```python
from build123d import *

# Parameters (mm, degrees)
BOSS_EXTRUDE1_DEPTH = 3.175
SKETCH2_R           = 1.5875
CUT_EXTRUDE1_DEPTH  = 64.286370995


with BuildPart() as part:
    # Sketch1 → Boss-Extrude1 (new body)
    with BuildSketch(Plane.XY):
        Polygon((40.909912505, -35.06563929), (40.909912505, -9.66563929), (-22.590087495, 41.13436071), (-47.990087495, 41.13436071), (-47.990087495, -35.06563929), align=None)
    extrude(amount=BOSS_EXTRUDE1_DEPTH)

    # Sketch2 → Cut-Extrude1 (cut, through all)
    with BuildSketch(Plane(origin=(0, 0, 0), x_dir=(-1, 0, 0), z_dir=(0, 0, -1))):
        with Locations((35.290087495, -22.36563929)):
            Circle(SKETCH2_R)
        with Locations((35.290087495, -3.31563929)):
            Circle(SKETCH2_R)
        with Locations((35.290087495, 15.73436071)):
            Circle(SKETCH2_R)
        with Locations((35.290087495, 34.78436071)):
            Circle(SKETCH2_R)
        with Locations((10.494914026, -22.36563929)):
            Circle(SKETCH2_R)
        with Locations((-8.555085974, -22.36563929)):
            Circle(SKETCH2_R)
        with Locations((-27.605085974, -22.36563929)):
            Circle(SKETCH2_R)
    extrude(amount=-CUT_EXTRUDE1_DEPTH, mode=Mode.SUBTRACT)


solid = part.part
```
Could you check a few things on this model? Use its own coordinates, in mm. Round coordinates to 2 decimals unless told otherwise and drop trailing zeros. Loops run counter-clockwise (first coordinate to the right, second up) from the corner with the lowest first, then second, coordinate; pieces in that order, holes last. Notation, with made-up numbers: M 11,82 L 37,82 A11 cw 37,103 Z; hole C 13.5,-8.5 d2. An arc over 180 degrees is marked long. Answer as CSV lines item,"result".
1) We'd pull the mould along X, two halves only. Please class faces 1 (the flat face through (40.91, -23, 2)), 2 (the cylindrical face through (8.899, -23.915, 1.565)), 3 (the flat face through (-4, -35.066, 2)), 4 (the cylindrical face through (-34.03, -4.28, 1.57)): released by +X, released by -X, zero draft, split by the parting line, or undercut.
From the geometry:
face 1,"released by +X"
face 2,"undercut"
face 3,"zero draft"
face 4,"undercut"
2) For pin 1 Ø3.5 at (x, y) = (-35.29, 34.78) entering from -Z, with a flat end and sliding along its axis, tell me the tip position at first contact or that it passes through.
From the geometry:
pin 1,"z = 0"
3) If I drill on probe 1 along Y at (x, z) = (-36, 2); probe 2 along Y at (x, z) = (29, 0.3); probe 3 along X at (y, z) = (33.5, 0.25), over which ranges is the centre line in solid material (lowest first)?
From the geometry:
probe 1,"-35.07 to -23.79, -20.95 to -4.74, -1.9 to 14.31, 17.15 to 33.36, 36.2 to 41.13"
probe 2,"-35.07 to -23.12, -21.61 to -0.14"
probe 3,"-47.99 to -36.22, -34.36 to -13.05"
4) Imagine slicing it at B-B on x = 35.5. List the corners of the cut face in (y, z) for me (3 decimals).
From the geometry:
outline,"M -35.066,0 L -5.338,0 L -5.338,3.175 L -35.066,3.175 Z"
5) Imagine slicing it at A-A on z = 1.1. List the corners of the cut face in (x, y) for me (1 decimal), and give its area (3 significant figures).
From the geometry:
outline,"M -48,-35.1 L 40.9,-35.1 L 40.9,-9.7 L -22.6,41.1 L -48,41.1 Z; hole C -35.3,-22.4 d3.2; hole C -35.3,-3.3 d3.2; hole C -35.3,15.7 d3.2; hole C -35.3,34.8 d3.2; hole C -10.5,-22.4 d3.2; hole C 8.6,-22.4 d3.2; hole C 27.6,-22.4 d3.2"
area,"5,110 mm^2"
6) Imagine slicing it at C-C on y = 7. List the corners of the cut face in (x, z) for me (3 decimals).
From the geometry:
outline,"M -47.99,0 L 20.078,0 L 20.078,3.175 L -47.99,3.175 Z"
